```python
from build123d import *

# Parameters (mm, degrees)
SKIZZE2_R                       = 1.55
SKIZZE2_W                       = 2.1
SKIZZE2_H                       = 6.2
AUFSATZ_LINEAR_AUSTRAGEN1_DEPTH = 10


with BuildPart() as part:
    # Skizze2 → Aufsatz-Linear austragen1 (new body)
    with BuildSketch(Plane(origin=(0, 0, -20.169507331), x_dir=(-1, 0, 0), z_dir=(0, 0, -1))):
        Polygon((-22.148061032, 15.226980034), (-19.148061032, 15.226980034), (-16.448061032, 15.226980034), (-16.148061032, 15.226980034), (-14.648061032, 15.226980034), (-14.648061032, 25.377216735), (-14.648061032, 32.226980034), (-19.148061032, 32.226980034), (-23.648061032, 32.226980034), (-23.648061032, 25.377216735), (-22.148061032, 25.377216735), align=None)
        with Locations((-19.148061032, 27.176743334)):
            Circle(SKIZZE2_R, mode=Mode.SUBTRACT)
        with Locations((-17.198061032, 20.288222167)):
            Rectangle(SKIZZE2_W, SKIZZE2_H, mode=Mode.SUBTRACT)
        with Locations((-20.196983303, 20.288222167)):
            Rectangle(SKIZZE2_W, SKIZZE2_H, mode=Mode.SUBTRACT)
    extrude(amount=AUFSATZ_LINEAR_AUSTRAGEN1_DEPTH)


solid = part.part
```
Design review of the part built by this model. Coordinates are the model's own, in mm. A direction names the side the tool comes from. Coordinates: 2 decimals unless noted, no trailing zeros. Write each loop counter-clockwise with the first axis right and the second up, starting at its lowest first coordinate (ties: lowest second). Pieces come first, ordered by that corner, then holes. Notation, with made-up numbers: M 67,-27.75 L 119,-27.75 A21 cw 119,-15.75 Z; hole C 49.25,16.25 d4. An arc over 180 degrees is marked long. Answer as a JSON object with one key per item and string values.
Item 1: Add section A-A, the plane y = 19.25. Give the boundary of the cut face in (x, z), and give its area (3 significant figures).
Outcome:
{"outline": "M 14.65,-30.17 L 16.15,-30.17 L 16.15,-20.17 L 14.65,-20.17 Z; M 18.25,-30.17 L 19.15,-30.17 L 19.15,-20.17 L 18.25,-20.17 Z; M 21.25,-30.17 L 22.15,-30.17 L 22.15,-20.17 L 21.25,-20.17 Z", "area": "33.0 mm²"}
Item 2: Machinability: for faces 4 (the flat face through (23.648, 29, -25)), 5 (the flat face through (19.147, 20, -25)), 6 (the flat face through (23, 25.377, -25)), which of the approach directions +Z, -Z, +X, -X, +Y, -Y give a long, thin tool a straight path to every point of the face, cutting with its end or side? Answer none if there is none.
Outcome:
{"face 4": "+Z, -Z, +X, +Y, -Y", "face 5": "+Z, -Z", "face 6": "+Z, -Z, +X, -Y"}
Item 3: Add section D-D, the plane y = 26. Give the boundary of the cut face in (x, z), and give its area (3 significant figures).
Outcome:
{"outline": "M 14.65,-30.17 L 18.14,-30.17 L 18.14,-20.17 L 14.65,-20.17 Z; M 20.16,-30.17 L 23.65,-30.17 L 23.65,-20.17 L 20.16,-20.17 Z", "area": "69.8 mm²"}
Item 4: Wall thickness on probe 1 along X at (y, z) = (22.25, -26.5); probe 2 along X at (y, z) = (24, -28.25); probe 3 along Y at (x, z) = (16.75, -26.75): over which ranges is each line inside the solid? List them lowest first.
Outcome:
{"probe 1": "14.65 to 16.15, 18.25 to 19.15, 21.25 to 22.15", "probe 2": "14.65 to 22.15", "probe 3": "15.23 to 17.19, 23.39 to 32.23"}
Item 5: Draft analysis for pull direction X (two halves, no side actions). For faces 1 (the flat face through (18.2, 25.7, -30.17)), 2 (the flat face through (22.148, 20, -25)), 3 (the flat face through (20, 17.188, -25)), state which applies: pulls with the +X half, pulls with the -X half, needs draft (parallel to the pull), parting line crosses it, or undercut.
Outcome:
{"face 1": "needs draft", "face 2": "pulls with the +X half", "face 3": "undercut"}
Item 6: Insertion check: pin 1 Ø4 at (x, y) = (20, 20) entering from +Z; pin 2 Ø5 at (y, z) = (19, -25) entering from +X. Each pin has a flat end and moves straight along its axis. Give the tip position at first contact, or say it passes through.
Outcome:
{"pin 1": "z = -20.17", "pin 2": "x = 22.15"}
Item 7: Add section B-B, the plane x = 16.75. Give the boundary of the cut face in (y, z).
Outcome:
{"outline": "M 15.23,-30.17 L 17.19,-30.17 L 17.19,-20.17 L 15.23,-20.17 Z; M 23.39,-30.17 L 32.23,-30.17 L 32.23,-20.17 L 23.39,-20.17 Z"}
Item 8: Add section C-C, the plane z = -21. Give the boundary of the cut face in (x, y).
Outcome:
{"outline": "M 14.65,15.23 L 22.15,15.23 L 22.15,25.38 L 23.65,25.38 L 23.65,32.23 L 14.65,32.23 Z; hole M 16.15,17.19 L 18.25,17.19 L 18.25,23.39 L 16.15,23.39 Z; hole C 19.15,27.18 d3.1; hole M 19.15,17.19 L 21.25,17.19 L 21.25,23.39 L 19.15,23.39 Z"}
